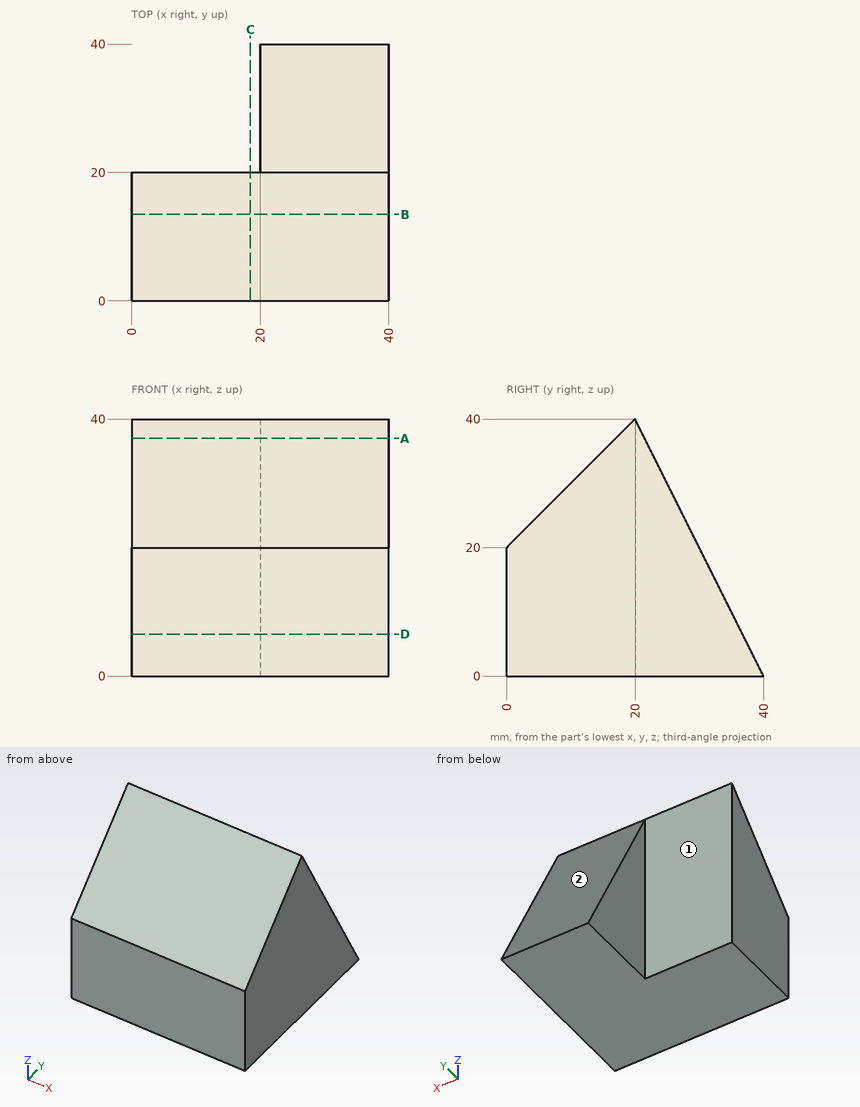
Design review of the part shown in the three views and the two pictorial views. Dimensions are in mm from the part's minimum x, y and z. A direction names the side the tool comes from. Round coordinates to 2 decimals unless told otherwise and drop trailing zeros. Order: outer loops, then holes, each group sorted by start corner. A loop starts at its lowest first (then second) coordinate and runs counter-clockwise, first axis right, second up. Notation, with made-up numbers: (-13, -2.75) - (43, -2.75) arc R8 cw to (43, 7.25) - close; hole circle Ø1 at (-22, 35.5). An arc over 180 degrees is marked (long way). Answer in a Markdown table with one row per item.
(1) Take a section at A-A on z = 37. Write out the cut boundary in (x, y), plus the area to 3 significant figures.
Result set:
| item | result |
|---|---|
| outline | (0, 17) - (40, 17) - (40, 21.5) - (20, 21.5) - (20, 20) - (0, 20) - close |
| area | 150 mm2 |
(2) Clearance check with flat-ended pins moving along their axes: P1, Ø6, axis at x = 30, y = 11.5, coming from the +Z side; P2, Ø2, axis at x = 4, z = 17, coming from the +Y side; P3, Ø10, axis at y = 31, z = 30, coming from the -X side; P4, Ø3, axis at y = 32, z = 10.5, coming from the -X side. State where each tip first meets the part, or that it passes through.
Result set:
| item | result |
|---|---|
| P1 | stops at z = 34.5 |
| P2 | stops at y = 20 |
| P3 | passes through |
| P4 | stops at x = 20 |
(3) Take a section at D-D on z = 6.5. Write out the cut boundary in (x, y), plus the area to 4 significant figures.
Result set:
| item | result |
|---|---|
| outline | (0, 0) - (40, 0) - (40, 36.75) - (20, 36.75) - (20, 20) - (0, 20) - close |
| area | 1,135 mm2 |
(4) Take a section at B-B on y = 13.5. Write out the cut boundary in (x, z), plus the area to 3 significant figures.
Result set:
| item | result |
|---|---|
| outline | (0, 0) - (40, 0) - (40, 33.5) - (0, 33.5) - close |
| area | 1,340 mm2 |
(5) For line 1 (X direction, y = 25, z = 7.5); line 2 (Y direction, x = 6.5, z = 4.5); line 3 (Y direction, x = 22.5, z = 4), list the stretches that pass through material, from the lowest coordinate up. Write a range as from..to.
Result set:
| item | result |
|---|---|
| line 1 | x = 20..40 |
| line 2 | y = 0..20 |
| line 3 | y = 0..38 |
(6) Take a section at C-C on x = 18.5. Write out the cut boundary in (y, z), plus the area to 3 significant figures.
Result set:
| item | result |
|---|---|
| outline | (0, 0) - (20, 0) - (20, 40) - (0, 20) - close |
| area | 600 mm2 |
(7) Machinability: for the marked faces 1 and 2, which of the approach directions +Z, -Z, +X, -X, +Y, -Y give a long, thin tool a straight path to every point of the face, cutting with its end or side? Answer none if there is none.
Result set:
| item | result |
|---|---|
| face 1 | +Z, -Z, -X, +Y |
| face 2 | +Z, +X, -X, +Y |
